Source: CAD feature listing. Evaluate the final solid. Frame: model axes, mm. Round coordinates to 2 decimals unless told otherwise and drop trailing zeros. Order: outer loops, then holes, each group sorted by start corner. A loop starts at its lowest first (then second) coordinate and runs counter-clockwise, first axis right, second up. Notation, with made-up numbers: (54.25, 59.25) - (108.25, 59.25) arc R26 cw to (108.25, 96.25) - close; hole circle Ø4 at (25, 51). An arc over 180 degrees is marked (long way). Use one line per item in the form item = value. Start each with the question number.
Q1. Cut plane D-D, the plane x = 6.5. Return the cut outline in (y, z), and give its area (3 significant figures).
Q2. Cut plane C-C, the plane x = 9. Return the cut outline in (y, z).
Q3. Ray query, line 1 (X direction, y = -3.1, z = -2.75); line 2 (X direction, y = -2.8, z = 2.75); line 3 (Z direction, x = 3.25, y = -4.1). Return the intervals inside material, ascending. Write a range as [from, to].
Q4. Cut plane A-A, the plane z = 1.25. Return the cut outline in (x, y), and give its area (3 significant figures).
Q5. Pin query (flat end, axial travel): pin 1 Ø3 at (x, y) = (7.5, -2) entering from +Z; pin 2 Ø1 at (y, z) = (-4.5, -0.5) entering from -X; pin 3 Ø1 at (y, z) = (-3, 3) entering from -X. Return the tip coordinate at first contact, or that it passes through.
Q6. Cut plane B-B, the plane y = -0.5. Give the number of separate pieces and of enclosed holes in the cut face, and give its area (3 significant figures).
from build123d import *

# Parameters (mm, degrees)
F0_R     = 0.325
F1_DEPTH = 5


# Not quite as in the source:
# - ends of sketch curves that miss each other by under 0.0002 mm in the source are joined


with BuildPart() as f1:
    # F0 (on Front) → F1 (new body)
    with BuildSketch(Plane.XZ):
        with BuildLine():
            Line((-11.295323, -2.696106), (-9.375, -3.81))
            ThreePointArc((-9.375, -3.81), (0, 1.590001), (9.3750005059, -3.8099997066))
            Line((9.3750005059, -3.8099997066), (11.295323, -2.696106))
            ThreePointArc((11.295323, -2.696106), (0, 3.810001), (-11.295323, -2.696106))
        make_face()
        with Locations((-8.873374, -0.467984)):
            Circle(F0_R, mode=Mode.SUBTRACT)
        with Locations((8.873374, -0.467984)):
            Circle(F0_R, mode=Mode.SUBTRACT)
        with Locations((-3.2525, 2.803828)):
            Circle(F0_R, mode=Mode.SUBTRACT)
        with Locations((3.2525, 2.803828)):
            Circle(F0_R, mode=Mode.SUBTRACT)
    extrude(amount=F1_DEPTH)


solid = f1.part
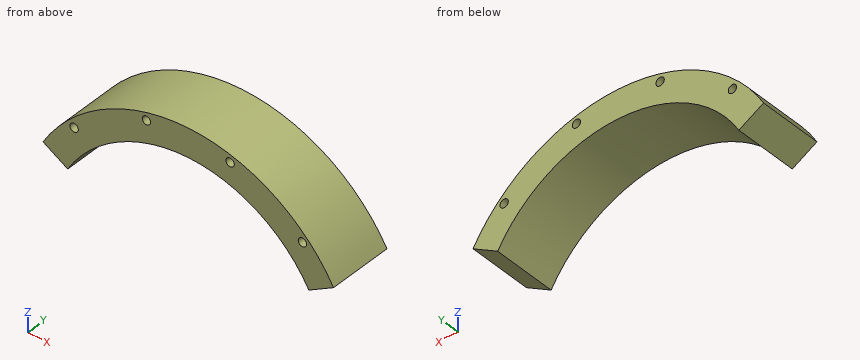
Completed:
q1.outline = (-5, -0.58) - (0, -0.58) - (0, 2.08) - (-5, 2.08) - close
q1.area = 13.3 mm2
q2.outline = (-5, -3.21) - (0, -3.21) - (0, -0.77) - (-5, -0.77) - close; (-5, -0.17) - (0, -0.17) - (0, 0.21) - (-5, 0.21) - close
q3.line_1 = [-11.2, -8.67], [8.67, 11.2]
q3.line_2 = [-5.15, -3.57], [-2.93, 2.93], [3.57, 5.15]
q3.line_3 = [1.09, 2.48], [3.13, 3.4]
q4.outline = (-7.77, -5) - (-2.69, -5) - (-2.69, 0) - (-7.77, 0) - close; (2.69, -5) - (7.77, -5) - (7.77, 0) - (2.69, 0) - close
q4.area = 50.7 mm2
q5.pin_1 = 2.35
q5.pin_2 = -10.12
q5.pin_3 = -5.7
q6.separate_pieces = 1
q6.enclosed_holes = 4
q6.area = 54.1 mm2
